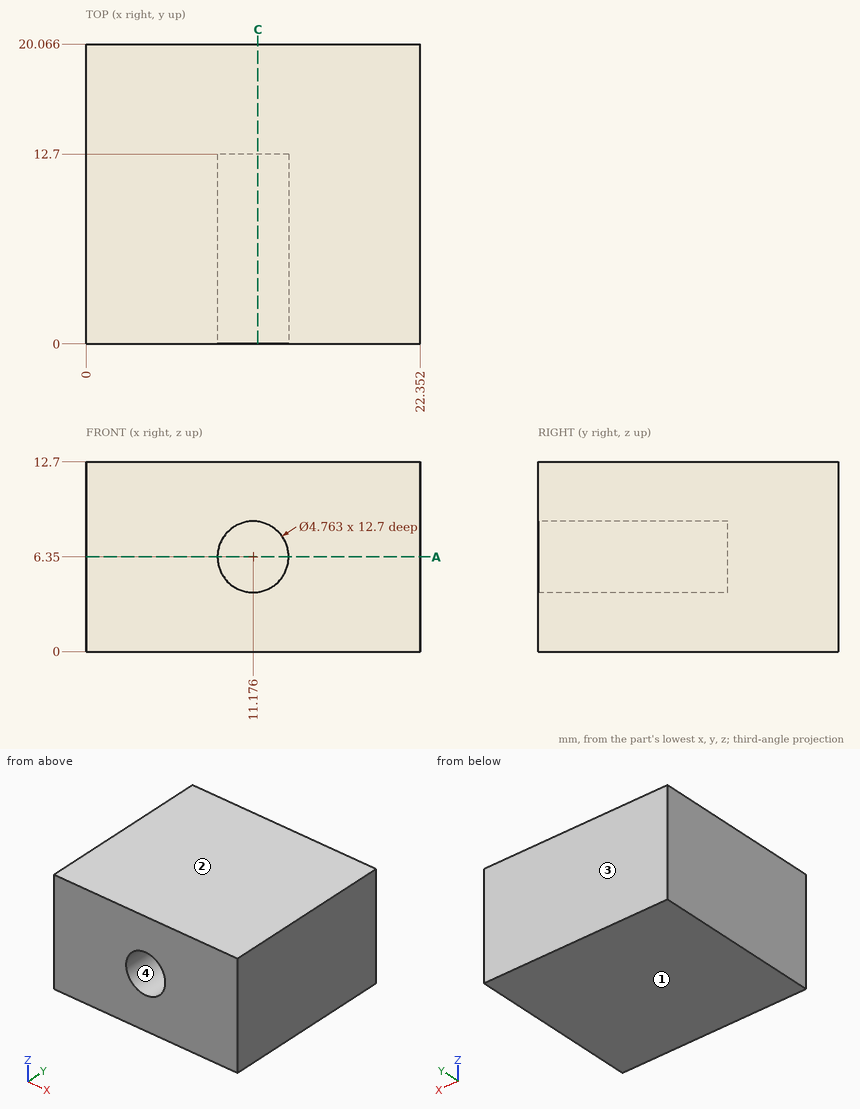
Input: dimensioned drawing with shaded views. Units: mm. Origin: part minimum x, y, z. Coordinates: 2 decimals unless noted, no trailing zeros. Loops run counter-clockwise (first coordinate to the right, second up) from the corner with the lowest first, then second, coordinate; pieces in that order, holes last. Notation, with made-up numbers: (77, 4) -> (88, 4) arc R21 cw to (88, 23) -> close; hole circle Ø6 at (69.5, 36). An arc over 180 degrees is marked (long way). Use a Markdown table: item, result. Add a question column.
(1) Pin query (flat end, axial travel): pin 1 Ø2.5 at (x, z) = (11.5, 6.5) entering from -Y. Return the tip coordinate at first contact, or that it passes through.
(2) Line query: line 1 along X through (y, z) = (7, 6.35) (1 decimal); line 2 along Z through (x, y) = (12.5, 4.5); line 3 along X through (y, z) = (5.5, 7) (1 decimal). Output: solid intervals per line, ascending.
(3) Section query C-C, the plane x = 11.5. Return loops of the section in (y, z) (1 decimal).
(4) Mould query, pull axis Z, two halves, no side actions, for the marked faces 1, 2, 3 and 4. Classes: pulls with the +Z half, pulls with the -Z half, needs draft (parallel to the pull), parting line crosses it, or undercut.
(5) Section query A-A, the plane z = 6.35. Return loops of the section in (x, y) (1 decimal).
Answer:
| question | item | result |
|---|---|---|
| 1 | pin 1 | stops at y = 12.7 |
| 2 | line 1 | x = 0 to 8.8, 13.6 to 22.4 |
| 2 | line 2 | z = 0 to 4.37, 8.33 to 12.7 |
| 2 | line 3 | x = 0 to 8.9, 13.5 to 22.4 |
| 3 | outline | (0, 0) -> (20.1, 0) -> (20.1, 12.7) -> (0, 12.7) -> (0, 8.7) -> (12.7, 8.7) -> (12.7, 4) -> (0, 4) -> close |
| 4 | face 1 | pulls with the -Z half |
| 4 | face 2 | pulls with the +Z half |
| 4 | face 3 | needs draft |
| 4 | face 4 | undercut |
| 5 | outline | (0, 0) -> (8.8, 0) -> (8.8, 12.7) -> (13.6, 12.7) -> (13.6, 0) -> (22.4, 0) -> (22.4, 20.1) -> (0, 20.1) -> close |
